Model file for the job. Use its own axes, mm. Face numbers are marked on the shaded views. A direction names the side the tool comes from. Round coordinates to 2 decimals unless told otherwise and drop trailing zeros. Write each loop counter-clockwise with the first axis right and the second up, starting at its lowest first coordinate (ties: lowest second). Pieces come first, ordered by that corner, then holes.
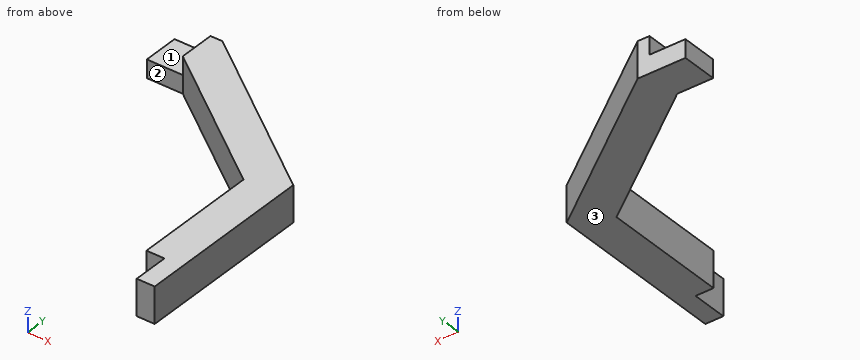
```python
from build123d import *

# Parameters (mm, degrees)
SALIENTE_EXTRUIR1_DEPTH = 20
CROQUIS2_W              = 20
CROQUIS2_H              = 20
CORTAR_EXTRUIR1_DEPTH   = 10
CROQUIS3_W              = 20
CROQUIS3_H              = 20
CORTAR_EXTRUIR2_DEPTH   = 10


with BuildPart() as part:
    # Croquis1 → Saliente-Extruir1 (new body)
    with BuildSketch(Plane.XY):
        Polygon((-60, 0), (-33.333333333, 0), (60, -70), (60, -170), (40, -170), (40, -80), (-40, -20), (-60, -20), align=None)
    extrude(amount=SALIENTE_EXTRUIR1_DEPTH)

    # Croquis2 → Cortar-Extruir1 (cut)
    with BuildSketch(Plane.XY.offset(20)):
        with Locations((-50, -10)):
            Rectangle(CROQUIS2_W, CROQUIS2_H)
    extrude(amount=-CORTAR_EXTRUIR1_DEPTH, mode=Mode.SUBTRACT)

    # Croquis3 → Cortar-Extruir2 (cut)
    with BuildSketch(Plane(origin=(40, 0, 0), x_dir=(0, 0, -1), z_dir=(1, 0, 0))):
        with Locations((-10, -160)):
            Rectangle(CROQUIS3_W, CROQUIS3_H)
    extrude(amount=CORTAR_EXTRUIR2_DEPTH, mode=Mode.SUBTRACT)


solid = part.part
```
1) Cut at B-B on y = -109.5. List the corners of the cut face in (x, z), and give its area (3 significant figures).
2) Cut at A-A on z = 11.75. List the corners of the cut face in (x, y), and give its area (3 significant figures).
3) Cut at C-C on x = -50. List the corners of the cut face in (y, z), and give its area (3 significant figures).
4) Cut at D-D on z = 3.25. List the corners of the cut face in (x, y), and give its area (3 significant figures).
5) Which spindle directions (+Z, -Z, +X, -X, +Y, -Y) get a long thin tool onto all of the face, cutting with end or side? Do the marked faces 1, 2 and 3. Say none if no direction does.
6) Wall check: probe 1 along X at (y, z) = (-97.5, 17); probe 2 along Y at (x, z) = (31, 13.5); probe 3 along Y at (x, z) = (-12.5, 11.5) (3 decimals). Give the ranges that are in metal, low to high.
7) Flat gauge pins, fed straight in: pin 1 Ø4 at (y, z) = (-46.5, 13) entering from +X; pin 2 Ø6 at (y, z) = (-22.5, 2.5) entering from +X; pin 3 Ø3 at (x, z) = (33.5, 14.5) entering from +Y. Where does each tip first touch, or does it go through?
Result sheet:
1. outline: (40, 0) - (60, 0) - (60, 20) - (40, 20) - close
1. area: 400 mm2
2. outline: (-40, -20) - (40, -80) - (40, -150) - (50, -150) - (50, -170) - (60, -170) - (60, -70) - (-33.33, 0) - (-40, 0) - close
2. area: 3,930 mm2
3. outline: (-20, 0) - (0, 0) - (0, 10) - (-20, 10) - close
3. area: 200 mm2
4. outline: (-60, -20) - (-40, -20) - (40, -80) - (40, -150) - (50, -150) - (50, -170) - (60, -170) - (60, -70) - (-33.33, 0) - (-60, 0) - close
4. area: 4,330 mm2
5. face 1: +Z, -X, +Y, -Y
5. face 2: +Z, -Z, -X, -Y
5. face 3: -Z, +X, -X, +Y, -Y
6. probe 1: x = 40 to 60
6. probe 2: y = -73.25 to -48.25
6. probe 3: y = -40.625 to -15.625
7. pin 1: stops at x = 31.33
7. pin 2: stops at x = 0.67
7. pin 3: stops at y = -49
